```python
from build123d import *

# Parameters (mm, degrees)
SKETCH_1_W          = 22
SKETCH_1_H          = 40
EXTRUDE_1_DEPTH     = 3
SKETCH_2_R          = 11
SKETCH_2_R_2        = 9.8
EXTRUDE_2_DEPTH     = 40
FILLET_1_R          = 1
SKETCH_3_W          = 16.462875958
SKETCH_3_H          = 8.59071229
CUT_EXTRUDE_1_DEPTH = 2


with BuildPart() as part:
    # Эскиз1 → Бобышка-Вытянуть1 (new body)
    with BuildSketch(Plane.XY):
        Rectangle(SKETCH_1_W, SKETCH_1_H)
    extrude(amount=EXTRUDE_1_DEPTH)

    # Эскиз2 → Бобышка-Вытянуть2 (add)
    with BuildSketch(Plane(origin=(0, 20, 0), x_dir=(1, 0, 0), z_dir=(0, 1, 0))):
        with Locations((0, -13.26772589)):
            Circle(SKETCH_2_R)
        with Locations(Location((0, -13.26772589, 0), (0, 0, 270))):
            Circle(SKETCH_2_R_2, mode=Mode.SUBTRACT)
    extrude(amount=-EXTRUDE_2_DEPTH)

    # Скругление1
    fillet_1_edges = [part.edges().sort_by_distance(p)[0] for p in [
        (-3.946366055, 0, 3),
        (3.946366055, 0, 3),
    ]]
    fillet(fillet_1_edges, radius=FILLET_1_R)

    # Эскиз3 → Вырез-Вытянуть1 (cut)
    with BuildSketch(Plane.XZ.offset(20)):
        Rectangle(SKETCH_3_W, SKETCH_3_H)
    extrude(amount=-CUT_EXTRUDE_1_DEPTH, mode=Mode.SUBTRACT)


solid = part.part
```
Input: part model. Units: mm. Frame: model coordinates. A direction names the side the tool comes from. Coordinates: 2 decimals unless noted, no trailing zeros. Write each loop counter-clockwise with the first axis right and the second up, starting at its lowest first coordinate (ties: lowest second). Pieces come first, ordered by that corner, then holes. Notation, with made-up numbers: M 67,-28 L 72,-28 A13 ccw 72,-22 Z; hole C 49,-39 d10. An arc over 180 degrees is marked long. Use one line per item in the form item = value.
Q1. Material intervals for probe 1 along X at (y, z) = (-18, 13); probe 2 along Z at (x, y) = (-7, 0.5); probe 3 along Y at (x, z) = (6.5, 3.75), sorted ascending. Write a range as from..to.
Answer below:
probe_1 = -11..-9.8, 9.8..11
probe_2 = 0..3.22, 4.78..6.41, 20.13..21.75
probe_3 = -18..20
Q2. Section A-A (x = 0). Return loops of the section in (y, z), plus the area to 3 significant figures.
Answer below:
outline = M -20,23.07 L 20,23.07 L 20,24.27 L -20,24.27 Z; M -18,0 L 20,0 L 20,3.47 L -18,3.47 Z
area = 180 mm²
Q3. First-contact query: pin 1 (4 mm diameter, centred on y = -12, z = 20.5, fed in from -X); pin 2 (1 mm diameter, centred on x = 6, y = -19.5, fed in from -Z); pin 3 (2 mm diameter, centred on x = -1.5, z = 1, fed in from -Y); pin 4 (10 mm diameter, centred on x = -2.5, z = 17, fed in from +Y). Flat tips, straight axial feed; report the tip coordinate or a pass-through.
Answer below:
pin_1 = -9.68
pin_2 = 4.3
pin_3 = -18
pin_4 = through
Q4. Draft query along Z for faces 1 (the face through (-8.231, -19, 1)), 2 (the face through (5, -19, 4.295)), 3 (the face through (-9, 0, 3)). Return one class per face: released by +Z, released by -Z, zero draft, split by the parting line, or undercut.
Answer below:
face_1 = zero draft
face_2 = released by -Z
face_3 = undercut
Q5. Section C-C (y = 2). Return loops of the section in (x, z), plus the area to 3 significant figures.
Answer below:
outline = M -11,0 L 11,0 L 11,3 L 7.62,3 A1 cw 6.99,4.77 A11 ccw long -6.99,4.77 A1 cw -7.62,3 L -11,3 Z; hole C 0,13.27 d19.6
area = 145 mm²
Q6. Section B-B (z = 7.75). Return loops of the section in (x, y), plus the area to 3 significant figures.
Answer below:
outline = M -9.52,-20 L -8.1,-20 L -8.1,20 L -9.52,20 Z; M 8.1,-20 L 9.52,-20 L 9.52,20 L 8.1,20 Z
area = 113 mm²
Q7. Set-up query: faces 4 (the face through (-11, 0, 1)), 5 (the face through (9, 0, 3)), 6 (the face through (0, -18, 2)), 7 (the face through (-5, -19, 4.295)). Return all of +Z, -Z, +X, -X, +Y, -Y with unobstructed straight access to the full face (end or side cutting, diameter ignored); none if empty.
Answer below:
face_4 = +Z, -Z, -X, +Y, -Y
face_5 = +X, +Y, -Y
face_6 = -Z, -Y
face_7 = -Z, +X, -X, -Y
